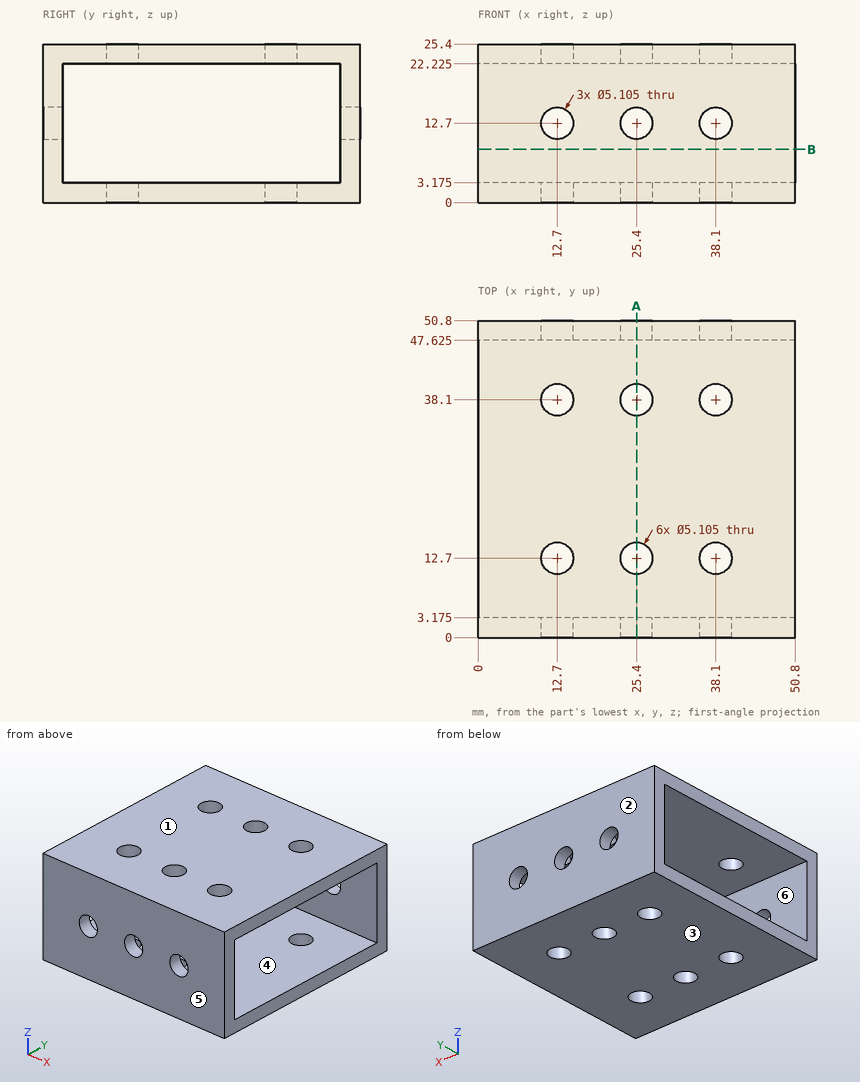
Print and shaded views of the part. All mm, measured from the part's lowest x, y and z. A direction names the side the tool comes from. Give positions to 0.01 mm unless a question says otherwise; leave off trailing zeros. Loops run counter-clockwise (first coordinate to the right, second up) from the corner with the lowest first, then second, coordinate; pieces in that order, holes last. Notation, with made-up numbers: (57.5, -36.75) -> (116.5, -36.75) arc R17 ccw to (116.5, -14.75) -> close; hole circle Ø9 at (-8, -37.75). An arc over 180 degrees is marked (long way). One line per question, with ' | ' between items. Start each with the question number.
1) Cut at A-A (x = 25.4). Count the separate pieces of the cut face and the enclosed holes in it, plus the area to 3 significant figures.
2) Pin check, flat tips, straight feed: pin 1 (4 mm diameter, centred on x = 25.4, z = 12.7, fed in from -Y); pin 2 (6 mm diameter, centred on x = 12.7, y = 38.1, fed in from +Z). Stop position of each tip, or through.
3) Cut at B-B (z = 8.5). Give the cut face in (x, y) (1 decimal).
4) Probe L1, parallel to Y at x = 12.7, z = 0.7; L2, parallel to Y at x = 28.5, z = 13.5 (1 decimal); L3, parallel to Z at x = 36, y = 28 (1 decimal). List the from-to ranges inside material, lowest first.
5) 3-axis set-ups, long thin cutter, end or side, ignore diameter. For the marked faces 5 and 6: which of +Z, -Z, +X, -X, +Y, -Y reach the whole face in a straight line?
6) Two-plate mould, pull along Z, no slides. Class the marked faces 1, 2, 3 and 4: released by +Z, released by -Z, zero draft, split by the parting line, or undercut.
Return value:
1) separate pieces: 6 | enclosed holes: 0 | area: 346 mm^2
2) pin 1: through | pin 2: z = 25.4
3) outline: (0, 0) -> (50.8, 0) -> (50.8, 3.2) -> (0, 3.2) -> close; (0, 47.6) -> (50.8, 47.6) -> (50.8, 50.8) -> (0, 50.8) -> close
4) L1: 0 to 10.15, 15.25 to 35.55, 40.65 to 50.8 | L2: 0 to 3.2, 47.6 to 50.8 | L3: 0 to 3.2, 22.2 to 25.4
5) face 5: +Z, -Z, +X, -X, -Y | face 6: +X, -X
6) face 1: released by +Z | face 2: zero draft | face 3: released by -Z | face 4: undercut
